from build123d import *

# Parameters (mm, degrees)
BOSS_EXTRUDE1_DEPTH = 3.175
FILLET1_R           = 27.78
SKETCH5_R           = 2
CUT_EXTRUDE2_DEPTH  = 95.405671522
SKETCH7_R           = 1.5
SKETCH7_R_2         = 3.925
CUT_EXTRUDE3_DEPTH  = 10


with BuildPart() as part:
    # Sketch1 → Boss-Extrude1 (new body)
    with BuildSketch(Plane(origin=(0, 0, 0), x_dir=(1, 0, 0), z_dir=(0, 1, 0))):
        Polygon((0, -94.945058207), (-86.602540378, 55.054941793), (86.602540378, 55.054941793), align=None)
    extrude(amount=BOSS_EXTRUDE1_DEPTH)

    # Fillet1
    fillet1_edges = [part.edges().sort_by_distance(p)[0] for p in [
        (0, 1.5875, 94.945058207),
        (-86.602540378, 1.5875, -55.054941793),
        (86.602540378, 1.5875, -55.054941793),
    ]]
    fillet(fillet1_edges, radius=FILLET1_R)

    # Sketch5 → Cut-Extrude2 (cut, through all)
    with BuildSketch(Plane(origin=(0, 3.175, 0), x_dir=(1, 0, 0), z_dir=(0, 1, 0))):
        with Locations(Location((32.5, 5.054941793, 0), (0, 0, 270))):
            Circle(SKETCH5_R)
        with Locations(Location((-32.5, 5.054941793, 0), (0, 0, 270))):
            Circle(SKETCH5_R)
        with Locations(Location((-10, 5.054941793, 0), (0, 0, 270))):
            Circle(SKETCH5_R)
        with Locations(Location((10, 5.054941793, 0), (0, 0, 270))):
            Circle(SKETCH5_R)
    extrude(amount=-CUT_EXTRUDE2_DEPTH, mode=Mode.SUBTRACT)

    # Sketch7 → Cut-Extrude3 (cut)
    with BuildSketch(Plane(origin=(0, 3.175, 0), x_dir=(1, 0, 0), z_dir=(0, 1, 0))):
        with Locations(Location((0, -30.885058207, 0), (0, 0, 270))):
            Circle(SKETCH7_R)
        with Locations(Location((-7.361215932, -43.635058207, 0), (0, 0, 270))):
            Circle(SKETCH7_R)
        with Locations(Location((0, -39.385058207, 0), (0, 0, 270))):
            Circle(SKETCH7_R_2)
        with Locations(Location((7.361215932, -43.635058207, 0), (0, 0, 270))):
            Circle(SKETCH7_R)
    extrude(amount=-CUT_EXTRUDE3_DEPTH, mode=Mode.SUBTRACT)


solid = part.part
Geometry: final body of the model. Coordinates: model frame, mm. Round coordinates to 2 decimals unless told otherwise and drop trailing zeros. Order: outer loops, then holes, each group sorted by start corner. A loop starts at its lowest first (then second) coordinate and runs counter-clockwise, first axis right, second up. Notation, with made-up numbers: (9.5, -30) -> (59.5, -30) arc R11 ccw to (59.5, -14) -> close; hole circle Ø9 at (74, 51.5). An arc over 180 degrees is marked (long way). Put each result on its own line as item: value. Start each with the question number.
Q1. Section A-A on x = 0. Return the cut outline in (y, z) (3 decimals), and give its area (3 significant figures).
Q2. Pull-direction query (X, two-part tool) for faces 1 (the cylindrical face through (30.548, 1.61, -5.489)), 2 (the flat face through (-43.032, 1.565, 20.412)), 3 (the flat face through (43.57, 1.57, 19.48)); classes: +X half, -X half, draft (parallel to the pull), parting line (faces both ways), or undercut.
Q3. Section B-B on y = 1.65. Give the number of separate pieces and of enclosed holes in the cut face, and give its area (3 significant figures).
Q4. Line query: probe 1 along X at (y, z) = (1.1, 43.5); probe 2 along X at (y, z) = (1.5, -5); probe 3 along Z at (x, y) = (41, 0.25). Output: solid intervals per line, ascending.
Q5. Section D-D on z = -10. Return the cut outline in (x, y) (3 decimals), and give its area (3 significant figures).
Q6. Section C-C on x = -32.5. Return the cut outline in (y, z) (3 decimals), and give its area (3 significant figures).
Ans:
1. outline: (0, -55.055) -> (3.175, -55.055) -> (3.175, 29.385) -> (0, 29.385) -> close; (0, 32.385) -> (3.175, 32.385) -> (3.175, 35.46) -> (0, 35.46) -> close; (0, 43.31) -> (3.175, 43.31) -> (3.175, 67.165) -> (0, 67.165) -> close
1. area: 354 mm2
2. face 1: undercut
2. face 2: -X half
2. face 3: +X half
3. separate pieces: 1
3. enclosed holes: 8
3. area: 11,300 mm2
4. probe 1: x = -29.7 to -8.86, -5.87 to 5.87, 8.86 to 29.7
4. probe 2: x = -57.7 to -34.5, -30.5 to -12, -8 to 8, 12 to 30.5, 34.5 to 57.7
4. probe 3: z = -54.94 to 23.93
5. outline: (-60.59, 0) -> (60.59, 0) -> (60.59, 3.175) -> (-60.59, 3.175) -> close
5. area: 385 mm2
6. outline: (0, -55.055) -> (3.175, -55.055) -> (3.175, -7.055) -> (0, -7.055) -> close; (0, -3.055) -> (3.175, -3.055) -> (3.175, 38.653) -> (0, 38.653) -> close
6. area: 285 mm2
